from build123d import *

# Parameters (mm, degrees)
F0_W      = 1651
F0_H      = 25.4
F1_DEPTH  = 152.4
F0_H_2    = 50.8
F2_DEPTH  = 25.4
F3_START  = 101.6
F2_FACE_W = 1651
F2_FACE_H = 50.8
F3_DEPTH  = 25.4


# Not quite as in the source:
# - a feature names something its author has since deleted; it is built from what else it names


with BuildPart() as f1:
    # F0 (on Front) → F1 (new body)
    with BuildSketch(Plane.XZ):
        Polygon((-850.9, 368.3), (-850.9, -393.7), (-825.5, -393.7), (-825.5, -12.7), (-825.5, 12.7), (-825.5, 317.5), (-825.5, 368.3), align=None)
        Polygon((-850.9, 393.7), (-850.9, 368.3), (-825.5, 368.3), (825.5, 368.3), (850.9, 368.3), (850.9, 393.7), align=None)
        Polygon((825.5, 12.7), (825.5, -12.7), (825.5, -393.7), (850.9, -393.7), (850.9, 368.3), (825.5, 368.3), (825.5, 317.5), align=None)
        Rectangle(F0_W, F0_H)
    extrude(amount=F1_DEPTH)

    # F0 (on Front) → F2 (join)
    with BuildSketch(Plane.XZ):
        with Locations((0, 342.9)):
            Rectangle(F0_W, F0_H_2)
    extrude(amount=F2_DEPTH)

    # F2_face (on face) → F3 (join)
    with BuildSketch(Plane(origin=(0, -25.4, 342.9), x_dir=(1, 0, 0), z_dir=(0, -1, 0)).offset(F3_START)):
        Rectangle(F2_FACE_W, F2_FACE_H)
    extrude(amount=F3_DEPTH)


solid = f1.part
The model under review builds one solid part; all positions refer to its coordinate system, in mm. A direction names the side the tool comes from. Round coordinates to 2 decimals unless told otherwise and drop trailing zeros. Write each loop counter-clockwise with the first axis right and the second up, starting at its lowest first coordinate (ties: lowest second). Pieces come first, ordered by that corner, then holes. Notation, with made-up numbers: M -17,44 L 21,44 A15 ccw 21,61 Z; hole C 7,-2.75 d3. An arc over 180 degrees is marked long. Use a Markdown table: item, result. Add a question column.
Q1. We need section A-A, the plane x = 595. State the section outline as (y, z) points.
Q2. The part is to be moulded in two halves that separate along X. For faces 4 (the face through (-12, -75, 12.7)), 5 (the face through (12, -75, 393.7)), 6 (the face through (850.9, -75, -6)), say which applies: pulls with the +X half, pulls with the -X half, needs draft (parallel to the pull), parting line crosses it, or undercut.
Q3. Machinability: for faces 1 (the face through (-67, 0, 323)), 2 (the face through (-12, -127, 343)), 3 (the face through (825.5, -75, -201)), which of the approach directions +Z, -Z, +X, -X, +Y, -Y give a long, thin tool a straight path to every point of the face, cutting with its end or side? Answer none if there is none.
Q4. To check wall thickness, follow line 1 (Z direction, x = 316, y = -28); line 2 (X direction, y = -46, z = 298); line 3 (Z direction, x = -613, y = -14). State the ranges of each line that lie inside material, in increasing order.
Q5. We need section C-C, the plane z = 214. State the section outline as (x, y) points, plus the area to 3 significant figures.
Q6. We need section B-B, the plane y = -45. State the section outline as (x, z) points, plus the area to 3 significant figures.
Q7. Insertion check: pin 1 (12.5 mm diameter, centred on x = 335, y = -138.5, fed in from -Z). The pin has a flat end and moves straight along its axis. Give the tip position at first contact, or say it passes through.
Findings below:
| question | item | result |
|---|---|---|
| 1 | outline | M -152.4,-12.7 L 0,-12.7 L 0,12.7 L -152.4,12.7 Z; M -152.4,317.5 L -127,317.5 L -127,368.3 L -25.4,368.3 L -25.4,317.5 L 0,317.5 L 0,393.7 L -152.4,393.7 Z |
| 2 | face 4 | undercut |
| 2 | face 5 | needs draft |
| 2 | face 6 | pulls with the +X half |
| 3 | face 1 | +Z, -Z, +X, -X, +Y |
| 3 | face 2 | none |
| 3 | face 3 | -Z, +Y, -Y |
| 4 | line 1 | z = -12.7 to 12.7, 368.3 to 393.7 |
| 4 | line 2 | x = -850.9 to -825.5, 825.5 to 850.9 |
| 4 | line 3 | z = -12.7 to 12.7, 317.5 to 393.7 |
| 5 | outline | M -850.9,-152.4 L -825.5,-152.4 L -825.5,0 L -850.9,0 Z; M 825.5,-152.4 L 850.9,-152.4 L 850.9,0 L 825.5,0 Z |
| 5 | area | 7,740 mm² |
| 6 | outline | M -850.9,-393.7 L -825.5,-393.7 L -825.5,-12.7 L 825.5,-12.7 L 825.5,-393.7 L 850.9,-393.7 L 850.9,393.7 L -850.9,393.7 Z; hole M -825.5,12.7 L 825.5,12.7 L 825.5,368.3 L -825.5,368.3 Z |
| 6 | area | 124,000 mm² |
| 7 | pin 1 | stops at z = -12.7 |
